Source: CAD feature listing. Evaluate the final solid. Frame: model axes, mm. A direction names the side the tool comes from. Round coordinates to 2 decimals unless told otherwise and drop trailing zeros. Order: outer loops, then holes, each group sorted by start corner. A loop starts at its lowest first (then second) coordinate and runs counter-clockwise, first axis right, second up. Notation, with made-up numbers: (79, -6.75) - (89, -6.75) arc R13 cw to (89, -1.75) - close; hole circle Ø11 at (-27.75, 56.5). An arc over 180 degrees is marked (long way). Put each result on its own line as item: value. Start each with the question number.
1) Section A-A on z = 3. Output: boundary loops of the cut face in (x, y).
2) Access query for faces 1 (the face through (14, 16, 6)), 2 (the face through (6, 10, 3)). Directions: +Z, -Z, +X, -X, +Y, -Y. A direction counts if a zero-diameter tool reaches every point of the face in a straight line with its end or side. Return the directions, or none.
3) Section B-B on x = 14. Output: boundary loops of the cut face in (y, z).
4) Contact query for flat-ended pins moving along their axis: P1, Ø1.5, axis at x = 10, z = 3, coming from the +Y side; P2, Ø1, axis at x = 5, z = 5.5, coming from the +Y side; P3, Ø3, axis at x = 6, z = 3, coming from the +Y side. Output: stop coordinate, or through.
5) Section D-D on z = 1.05. Output: boundary loops of the cut face in (x, y), then the cut area to 3 significant figures.
6) Line query: probe 1 along X at (y, z) = (5.5, 3); probe 2 along Z at (x, y) = (22, 6.5); probe 3 along Y at (x, z) = (14, 4.45). Output: solid intervals per line, ascending. Write a range as [from, to].
7) Mould query, pull axis X, two halves, no side actions, for faces 3 (the face through (22, 10, 3)), 4 (the face through (14, 0, 3)), 5 (the face through (14, 32, 3)). Classes: +X half, -X half, draft (parallel to the pull), parting line (faces both ways), or undercut.
8) Section C-C on x = 22. Output: boundary loops of the cut face in (y, z).
```python
from build123d import *

# Parameters (mm, degrees)
ESQUISSE1_W             = 28
ESQUISSE1_H             = 32
BOSS_EXTRU_1_DEPTH      = 6
ESQUISSE2_R             = 1.25
ENL_V_MAT_EXTRU_1_DEPTH = 10
ESQUISSE3_R             = 1.25
ENL_V_MAT_EXTRU_2_DEPTH = 43.941821107
ENL_V_MAT_EXTRU_3_DEPTH = 43.941821107


with BuildPart() as part:
    # Esquisse1 → Boss.-Extru.1 (new body)
    with BuildSketch(Plane.XY):
        with Locations((14, 16)):
            Rectangle(ESQUISSE1_W, ESQUISSE1_H)
    extrude(amount=BOSS_EXTRU_1_DEPTH)

    # Esquisse2 → Enlèv. mat.-Extru.1 (cut)
    with BuildSketch(Plane.XZ):
        with Locations(Location((6, 3, 0), (0, 0, 270))):
            Circle(ESQUISSE2_R)
        with Locations(Location((22, 3, 0), (0, 0, 90))):
            Circle(ESQUISSE2_R)
    extrude(amount=-ENL_V_MAT_EXTRU_1_DEPTH, mode=Mode.SUBTRACT)

    # Esquisse3 → Enlèv. mat.-Extru.2 (cut, through all)
    with BuildSketch(Plane.XY.offset(6)):
        with Locations((14, 19)):
            Circle(ESQUISSE3_R)
    extrude(amount=-ENL_V_MAT_EXTRU_2_DEPTH, mode=Mode.SUBTRACT)

    # Esquisse5 → Enlèv. mat.-Extru.3 (cut, through all)
    with BuildSketch(Plane.XY.offset(6)):
        with BuildLine():
            Line((0, 19), (0, 33))
            Line((0, 33), (28, 33))
            Line((28, 33), (28, 19))
            ThreePointArc((28, 19), (14, 32), (0, 19))
        make_face()
    extrude(amount=-ENL_V_MAT_EXTRU_3_DEPTH, mode=Mode.SUBTRACT)


solid = part.part
```
Answer sheet:
1. outline: (0, 0) - (4.75, 0) - (4.75, 10) - (7.25, 10) - (7.25, 0) - (20.75, 0) - (20.75, 10) - (23.25, 10) - (23.25, 0) - (28, 0) - (28, 19) arc R14.04 ccw to (0, 19) - close; hole circle Ø2.5 at (14, 19)
2. face 1: +Z, +X, -X, +Y, -Y
2. face 2: -Y
3. outline: (0, 0) - (17.75, 0) - (17.75, 6) - (0, 6) - close; (20.25, 0) - (32, 0) - (32, 6) - (20.25, 6) - close
4. P1: y = 31.62
4. P2: y = 29.13
4. P3: y = 30.4
5. outline: (0, 0) - (28, 0) - (28, 19) arc R14.04 ccw to (0, 19) - close; hole circle Ø2.5 at (14, 19)
5. area: 808 mm^2
6. probe 1: [0, 4.75], [7.25, 20.75], [23.25, 28]
6. probe 2: [0, 1.75], [4.25, 6]
6. probe 3: [0, 17.75], [20.25, 32]
7. face 3: undercut
7. face 4: draft
7. face 5: parting line
8. outline: (0, 0) - (29.5, 0) - (29.5, 6) - (0, 6) - (0, 4.25) - (10, 4.25) - (10, 1.75) - (0, 1.75) - close
